```python
from build123d import *

# Parameters (mm, degrees)
SKETCH1_R           = 6
BOSS_EXTRUDE1_DEPTH = 10


with BuildPart() as part:
    # Sketch1 → Boss-Extrude1 (new, symmetric)
    with BuildSketch(Plane(origin=(0, 0, 0), x_dir=(0, 0, -1), z_dir=(1, 0, 0))):
        with BuildLine():
            Line((12.5, -17.5), (-12.5, -17.5))
            ThreePointArc((-12.5, -17.5), (-30, 0), (-12.5, 17.5))
            Line((-12.5, 17.5), (12.5, 17.5))
            ThreePointArc((12.5, 17.5), (30, 0), (12.5, -17.5))
        make_face()
        Circle(SKETCH1_R, mode=Mode.SUBTRACT)
    extrude(amount=BOSS_EXTRUDE1_DEPTH, both=True)


solid = part.part
```
Could you check a few things on this model? Use its own coordinates, in mm. Give positions to 0.01 mm unless a question says otherwise; leave off trailing zeros. Loops run counter-clockwise (first coordinate to the right, second up) from the corner with the lowest first, then second, coordinate; pieces in that order, holes last. Notation, with made-up numbers: (20.25, 64.5) - (33.25, 64.5) arc R30 ccw to (33.25, 91.5) - close; hole circle Ø10 at (41.5, 15). An arc over 180 degrees is marked (long way). Use one line per item in the form item = value.
1. I want a section at C-C (y = -7). Please give me the cut outline in (x, z).
Response values:
outline = (-10, -28.54) - (10, -28.54) - (10, 28.54) - (-10, 28.54) - close
2. I want a section at A-A (y = 0). Please give me the cut outline in (x, z), and give its area (3 significant figures).
Response values:
outline = (-10, -30) - (10, -30) - (10, -6) - (-10, -6) - close; (-10, 6) - (10, 6) - (10, 30) - (-10, 30) - close
area = 960 mm²
3. I need wall thicknesses on probe 1 along Y at (x, z) = (-5.5, 0); probe 2 along Z at (x, y) = (-4.75, -1); probe 3 along Z at (x, y) = (-1.5, 1.5). Which ranges of each line are inside material? Lowest first, please.
Response values:
probe_1 = -17.5 to -6, 6 to 17.5
probe_2 = -29.97 to -5.92, 5.92 to 29.97
probe_3 = -29.94 to -5.81, 5.81 to 29.94
4. I want a section at B-B (x = 1.75). Please give me the cut outline in (y, z).
Response values:
outline = (-17.5, -12.5) arc R17.5 ccw to (17.5, -12.5) - (17.5, 12.5) arc R17.5 ccw to (-17.5, 12.5) - close; hole circle Ø12 at (0, 0)
5. Thinking about a two-plate mould opening in Y: for faces 1 (the face through (-10, 0.2, 6.2)), 2 (the face through (0, 0, -30)), 3 (the face through (0, 0, 6)), which applies, released by +Y, released by -Y, zero draft, split by the parting line, or undercut?
Response values:
face_1 = zero draft
face_2 = split by the parting line
face_3 = undercut
6. I want a section at D-D (z = -19). Please give me the cut outline in (x, y).
Response values:
outline = (-10, -16.25) - (10, -16.25) - (10, 16.25) - (-10, 16.25) - close
7. I'm going to push flat-ended pins straight in: pin 1 Ø1.5 at (x, y) = (1.5, 8) entering from +Z; pin 2 Ø4 at (x, y) = (0, -7.5) entering from +Z; pin 3 Ø10 at (x, z) = (2, -21) entering from -Y. Where does each tip first touch, or does it pass through?
Response values:
pin_1 = 28.43
pin_2 = 29.11
pin_3 = -17.15
